```python
from build123d import *

# Parameters (mm, degrees)
SKETCH1_R           = 2.8
BOSS_EXTRUDE1_DEPTH = 19.5
CUT_EXTRUDE1_DEPTH  = 8
SKETCH3_R           = 1
CUT_EXTRUDE2_DEPTH  = 6
SKETCH5_R           = 7
BOSS_EXTRUDE2_DEPTH = 5
SKETCH7_R           = 2.9
SKETCH7_R_2         = 2.6
CUT_EXTRUDE3_DEPTH  = 19.5


with BuildPart() as part:
    # Sketch1 → Boss-Extrude1 (new, symmetric)
    with BuildSketch(Plane(origin=(0, 0, 0), x_dir=(0, 0, -1), z_dir=(1, 0, 0))):
        Circle(SKETCH1_R)
    extrude(amount=BOSS_EXTRUDE1_DEPTH, both=True)

    # Sketch2 → Cut-Extrude1 (cut)
    with BuildSketch(Plane(origin=(19.5, 0, 0), x_dir=(0, 0, -1), z_dir=(1, 0, 0))):
        with BuildLine():
            Line((-1.85, 2.101784956), (-1.85, -2.101784956))
            ThreePointArc((-1.85, -2.101784956), (-2.8, 0), (-1.85, 2.101784956))
        make_face()
        with BuildLine():
            Line((1.85, 2.101784956), (1.85, -2.101784956))
            ThreePointArc((1.85, -2.101784956), (2.8, 0), (1.85, 2.101784956))
        make_face()
    extrude(amount=-CUT_EXTRUDE1_DEPTH, mode=Mode.SUBTRACT)

    # Sketch3 → Cut-Extrude2 (cut)
    with BuildSketch(Plane(origin=(19.5, 0, 0), x_dir=(0, 0, -1), z_dir=(1, 0, 0))):
        Circle(SKETCH3_R)
    extrude(amount=-CUT_EXTRUDE2_DEPTH, mode=Mode.SUBTRACT)

    # Sketch5 → Boss-Extrude2 (add)
    with BuildSketch(Plane.ZY.offset(19.5)):
        Circle(SKETCH5_R)
    extrude(amount=BOSS_EXTRUDE2_DEPTH)

    # Sketch7 → Cut-Extrude3 (cut)
    with BuildSketch(Plane(origin=(0, 0, 0), x_dir=(0, 0, -1), z_dir=(1, 0, 0))):
        Circle(SKETCH7_R)
        Circle(SKETCH7_R_2, mode=Mode.SUBTRACT)
    extrude(amount=-CUT_EXTRUDE3_DEPTH, mode=Mode.SUBTRACT)


solid = part.part
```
Read the model definition and answer for the solid it produces. Units are mm, in the model's axes. A direction names the side the tool comes from. Coordinates: 2 decimals unless noted, no trailing zeros. Loops run counter-clockwise (first coordinate to the right, second up) from the corner with the lowest first, then second, coordinate; pieces in that order, holes last. Notation, with made-up numbers: (-19, -29) -> (8, -29) arc R29 ccw to (8, 8) -> close; hole circle Ø1 at (87, 78). An arc over 180 degrees is marked (long way). Return JSON: item names as keys, results as strings.
Item 1: Find section C-C (x = 4.5). Determine the outline of the cut face in (y, z).
Answers:
{"outline": "circle Ø5.6 at (0, 0)"}
Item 2: Find the intervals of material crossed by probe 1 along Y at (x, z) = (18.2, 0); probe 2 along X at (y, z) = (0.75, -4.75); probe 3 along Z at (x, y) = (14.5, 1.5), in increasing order.
Answers:
{"probe 1": "y = -2.8 to -1, 1 to 2.8", "probe 2": "x = -24.5 to -19.5", "probe 3": "z = -1.85 to 1.85"}
Item 3: Flat-ended cylindrical pins translate along their axes: P1, Ø1.5, axis at x = 10.5, y = 1, coming from the -Z side; P2, Ø1, axis at y = -1, z = -2.5, coming from the +X side; P3, Ø2, axis at x = 15, y = -0.5, coming from the -Z side. Find the tip coordinate at first contact, or state that the pin passes through.
Answers:
{"P1": "stops at z = -2.79", "P2": "stops at x = 11.5", "P3": "stops at z = -1.85"}
Item 4: Find section B-B (y = 0). Determine the outline of the cut face in (x, z).
Answers:
{"outline": "(-24.5, -7) -> (-19.5, -7) -> (-19.5, -2.6) -> (0, -2.6) -> (0, -2.8) -> (11.5, -2.8) -> (11.5, -1.85) -> (19.5, -1.85) -> (19.5, -1) -> (13.5, -1) -> (13.5, 1) -> (19.5, 1) -> (19.5, 1.85) -> (11.5, 1.85) -> (11.5, 2.8) -> (0, 2.8) -> (0, 2.6) -> (-19.5, 2.6) -> (-19.5, 7) -> (-24.5, 7) -> close"}
Item 5: For faces 5 (the flat face through (16, 0, 1.85)), 6 (the flat face through (13.5, 0, 0)), 7 (the cylindrical face through (-9.614, 2.578, 0.338)), determine the directions among +Z, -Z, +X, -X, +Y, -Y from which every point of the face is accessible in a straight line to the end or side of a thin tool.
Answers:
{"face 5": "+Z, +X, +Y, -Y", "face 6": "+X", "face 7": "none"}
Item 6: Find section D-D (x = -12.5). Determine the outline of the cut face in (y, z).
Answers:
{"outline": "circle Ø5.2 at (0, 0)"}
Item 7: Find section A-A (z = 0). Determine the outline of the cut face in (x, y), plus the area to 3 significant figures.
Answers:
{"outline": "(-24.5, -7) -> (-19.5, -7) -> (-19.5, -2.6) -> (0, -2.6) -> (0, -2.8) -> (19.5, -2.8) -> (19.5, -1) -> (13.5, -1) -> (13.5, 1) -> (19.5, 1) -> (19.5, 2.8) -> (0, 2.8) -> (0, 2.6) -> (-19.5, 2.6) -> (-19.5, 7) -> (-24.5, 7) -> close", "area": "269 mm2"}
Item 8: For a pull along Z with two mould halves and no side action, classify faces 1 (the flat face through (19.5, -1, 1)), 2 (the cylindrical face through (7.72, -1.072, -2.586)), 3 (the flat face through (16, 0, -1.85)), 4 (the cylindrical face through (17, -1, 0)) as +Z half, -Z half, draft (parallel to the pull), parting line (faces both ways), or undercut.
Answers:
{"face 1": "draft", "face 2": "parting line", "face 3": "-Z half", "face 4": "undercut"}
